Source: three-view drawing plus pictorial views. Frame: mm from the lowest corner of the part. Give positions to 0.01 mm unless a question says otherwise; leave off trailing zeros. Loops run counter-clockwise (first coordinate to the right, second up) from the corner with the lowest first, then second, coordinate; pieces in that order, holes last. Notation, with made-up numbers: (-33, 75.25) -> (-17, 75.25) arc R20 ccw to (-17, 107.25) -> close; hole circle Ø8 at (-3, 65). An arc over 180 degrees is marked (long way). Put each result on its own line as item: value.
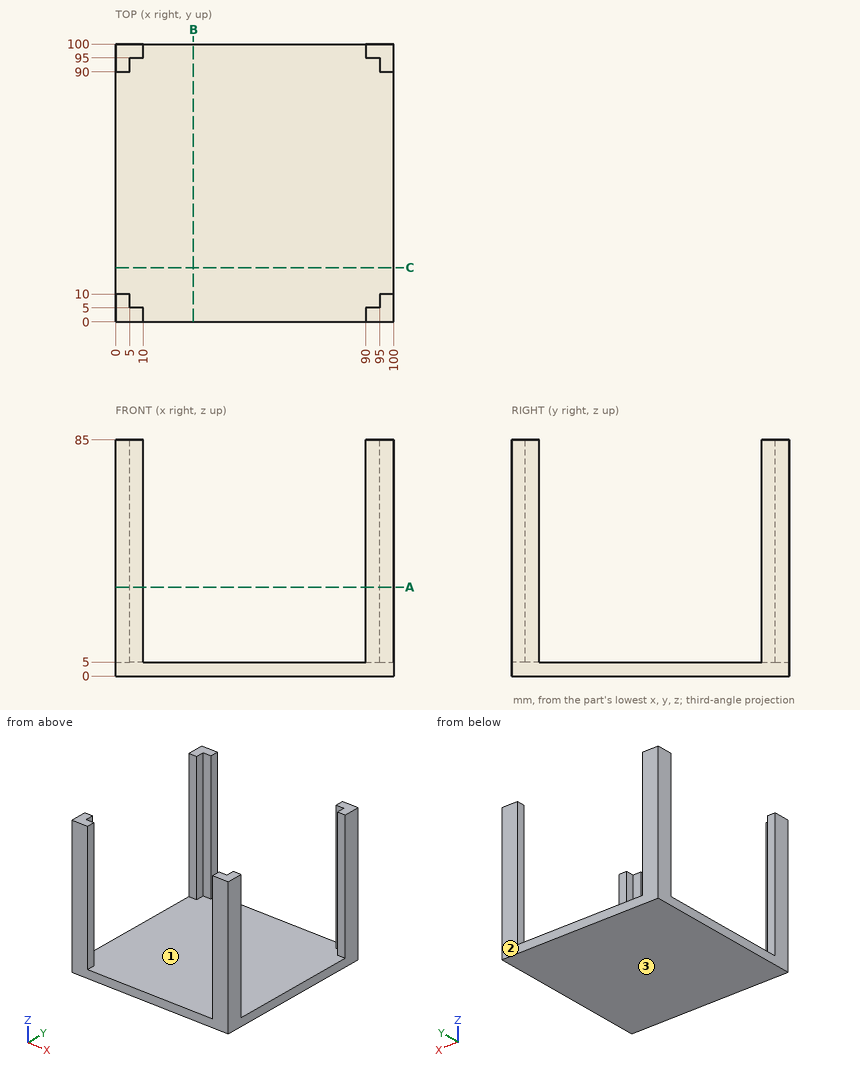
(1) Section B-B on x = 28. Return loops of the section in (y, z), then the cut area to 3 significant figures.
Calculated:
outline: (0, 0) -> (100, 0) -> (100, 5) -> (0, 5) -> close
area: 500 mm²
(2) Section A-A on z = 32. Return loops of the section in (x, y).
Calculated:
outline: (0, 0) -> (10, 0) -> (10, 5) -> (5, 5) -> (5, 10) -> (0, 10) -> close; (0, 90) -> (5, 90) -> (5, 95) -> (10, 95) -> (10, 100) -> (0, 100) -> close; (90, 0) -> (100, 0) -> (100, 10) -> (95, 10) -> (95, 5) -> (90, 5) -> close; (90, 95) -> (95, 95) -> (95, 90) -> (100, 90) -> (100, 100) -> (90, 100) -> close
(3) First-contact query: P1, Ø1.5, axis at x = 97.5, z = 55.5, coming from the -Y side; P2, Ø2, axis at x = 33.5, y = 12, coming from the +Z side; P3, Ø12, axis at y = 79, z = 30.5, coming from the +X side. Flat tips, straight axial feed; report the tip coordinate or a pass-through.
Calculated:
P1: stops at y = 0
P2: stops at z = 5
P3: passes through
(4) Draft query along Y for the marked faces 1, 2 and 3. Return one class per face: released by +Y, released by -Y, zero draft, split by the parting line, or undercut.
Calculated:
face 1: undercut
face 2: released by +Y
face 3: zero draft
(5) Line query: probe 1 along X at (y, z) = (8, 73); probe 2 along Z at (x, y) = (40.5, 14.5). Output: solid intervals per line, ascending. Write a range as from..to.
Calculated:
probe 1: x = 0..5, 95..100
probe 2: z = 0..5
